Model file for the job. Use its own axes, mm. Give positions to 0.01 mm unless a question says otherwise; leave off trailing zeros. Loops run counter-clockwise (first coordinate to the right, second up) from the corner with the lowest first, then second, coordinate; pieces in that order, holes last. Notation, with made-up numbers: (87.25, -18.75) - (97.25, -18.75) arc R22 cw to (97.25, 8.25) - close; hole circle Ø5 at (67.25, 51). An arc over 180 degrees is marked (long way). Use a Markdown table: item, result.
Autodesk Inventor part; units mm, degrees
ref_plane "YZ Plane" through (0, 0, 0) normal (1, 0, 0) x (0, 1, 0)
ref_plane "XZ Plane" through (0, 0, 0) normal (0, 1, 0) x (-1, 0, 0)
ref_plane "XY Plane" through (0, 0, 0) normal (0, 0, 1) x (1, 0, 0)
sketch "Sketch1" plane through (0, 0, 0) normal (0, 0, 1) x (1, 0, 0)
  arc A0 (-4.9984, 0.1266) -> (-4.98, 0.4466) centre (0, 0) ccw
  circle A1 centre (0, 0) radius 7.5
  circle A2 centre (0, 0) radius 7
  circle A3 centre (0, 0) radius 7
  point P0 (0, 0)
extrude "Extrusion1" add sketch "Sketch1" along normal blind 6 contours A2
sketch "Sketch2" plane through (0, 0, 6) normal (0, 0, 1) x (1, 0, 0)
  line L0 (0, 0) -> (-2.839, 0)
  line L1 (-2.839, 0) -> (-2.839, 2.1073)
  line L2 (-2.839, 2.1073) -> (0, 2.1073)
  line L3 (0, 2.1073) -> (0, 0)
extrude "Extrusion2" add sketch "Sketch2" along normal blind 1
sketch "Sketch3" plane through (0, 0, 6) normal (1, 0, 0) x (0, 0, -1)
  line L0 (0, 7) -> (0, -7)
  line L1 (0, 2.1073) -> (0, 0)
  line L2 (0, 0) -> (-1, 0)
  arc A0 (0, 0) -> (-5.1393, -1.322) centre (-0.5, -8.7067) ccw
  point P0 (6, 0)
  point P1 (-3.7243, -0.9054)
  point P2 (-4.3276, -1.2024)
sketch "Sketch4" plane through (0, 0, 6) normal (0, 0, 1) x (1, 0, 0)
  circle A0 centre (0, 0) radius 7
  circle A1 centre (0, 0) radius 2.65
  dimension "d20" = 5.3
sketch "Sketch8" plane through (0, 0, 7) normal (0, 0, 1) x (1, 0, 0)
  circle A0 centre (0, 0) radius 2.65
  dimension "d17" = 5.3
extrude "Extrusion3" cut sketch "Sketch8" against normal blind 100
sweep "Sweep6" add profiles "Sketch4" path "Sketch3" path curves A0
fillet "Fillet2" radius 2 2 edges at (-2.65, -1.322, 11.1393) (-7, -1.322, 11.1393)
properties part number "Eyes"
(1) Mould opens along X. For faces 1 (the flat face through (0, -3, 0)), 2 (the cylindrical face through (6.466, 2.681, 2.958)), 3 (the cylindrical face through (-2.647, 0.117, 3.549)) say: pulls with the +X half, pulls with the -X half, needs draft (parallel to the pull), parting line crosses it, or undercut.
Computed:
| item | result |
|---|---|
| face 1 | needs draft |
| face 2 | parting line crosses it |
| face 3 | undercut |
(2) Slice it at A-A, the plane z = 3.25. Write the cut outline in (x, y), plus the area to 3 significant figures.
Computed:
| item | result |
|---|---|
| outline | circle Ø14 at (0, 0); hole circle Ø5.3 at (0, 0) |
| area | 132 mm² |
(3) Drill centre lines: probe 1 along Y at (x, z) = (0, 5); probe 2 along X at (y, z) = (-1, 9.5); probe 3 along Z at (x, y) = (-3.75, 4). Where is each one in solid material? Low to high. Write a range as [from, to].
Computed:
| item | result |
|---|---|
| probe 1 | [-7, -2.65], [2.65, 7] |
| probe 2 | [-6.93, -2.69], [2.69, 6.93] |
| probe 3 | [0, 13.24] |
(4) Pin check, flat tips, straight feed: P1, Ø2, axis at x = 0, z = 12, coming from the -Y side; P2, Ø1.5, axis at x = 0.5, y = -4, coming from the +Z side; P3, Ø5, axis at y = -1, z = 12, coming from the +X side. Stop position of each tip, or through.
Computed:
| item | result |
|---|---|
| P1 | y = 1.3 |
| P2 | z = 8.51 |
| P3 | x = 6.99 |
